The model under review builds one solid part; all positions refer to its coordinate system, in mm. A direction names the side the tool comes from. Round coordinates to 2 decimals unless told otherwise and drop trailing zeros. Order: outer loops, then holes, each group sorted by start corner. A loop starts at its lowest first (then second) coordinate and runs counter-clockwise, first axis right, second up. Notation, with made-up numbers: M -10,74.25 L 48,74.25 A27 ccw 48,100.25 Z; hole C 68,4 d11. An arc over 180 degrees is marked long. Answer as a JSON object with one key per item and string values. Group by question number.
1) Consider section A-A, the plane z = 0. Write out the cut boundary in (x, y), then the cut area to 3 significant figures.
2) For faces 1 (the flat face through (0, 26, 4.5)), 2 (the flat face through (1.05, 1, -5)), 3 (the flat face through (-0.1, 5, 18.2)), list the 3-axis set-ups (+Z, -Z, +X, -X, +Y, -Y) from which the entire face can be reached by the end or side of a thin tool; tool diameter is ignored.
3) Consider section B-B, the plane y = 16. Write out the cut boundary in (x, z), then the cut area to 3 significant figures.
4) Consider section C-C, the plane z = -14. Write out the cut boundary in (x, y).
5) The part is to be moulded in two halves that separate along Z. For faces 4 (the flat face through (6.5, 2.5, -19.5)), 5 (the cylindrical face through (0, 4, -18)), 6 (the flat face through (-6.5, 2.5, 19.5)), say which applies: +Z half, -Z half, draft (parallel to the pull), parting line (faces both ways), or undercut.
6) To check wall thickness, follow line 1 (Z direction, x = 0, y = 2.35); line 2 (Z direction, x = 0, y = 1.1); line 3 (Z direction, x = 0, y = 3.75). State the ranges of each line that lie inside material, in increasing order.
7) Insertion check: pin 1 Ø5.5 at (x, z) = (-1.5, -16) entering from +Y; pin 2 Ø1 at (x, z) = (0, -4.5) entering from -Y; pin 3 Ø1.5 at (x, y) = (0.5, 7) entering from +Z; pin 4 Ø4 at (x, z) = (0, 14) entering from +Y. Each pin has a flat end and moves straight along its axis. Give the tip position at first contact, or say it passes through.
Autodesk Inventor part; units mm, degrees
ref_plane "YZ Plane" through (0, 0, 0) normal (1, 0, 0) x (0, 1, 0)
ref_plane "XZ Plane" through (0, 0, 0) normal (0, 1, 0) x (-1, 0, 0)
ref_plane "XY Plane" through (0, 0, 0) normal (0, 0, 1) x (1, 0, 0)
sketch "Sketch1" plane through (0, 0, 0) normal (0, 1, 0) x (-1, 0, 0)
  line L0 (7, 9) -> (-7, 9)
  line L1 (-7, 9) -> (-7, -9)
  line L2 (-7, -9) -> (7, -9)
  line L3 (7, -9) -> (7, 9)
  line L4 (7, 9) -> (-7, -9) construction
  line L5 (-7, 9) -> (7, -9) construction
  point P0 (0, 0)
  dimension "POST_WIDTH" = 18
  dimension "POST_LENGTH" = 14
extrude "Extrusion1" add sketch "Sketch1" along normal blind 28.05
sketch "Sketch2" plane through (0, 0, 0) normal (0, -1, 0) x (1, 0, 0)
  line L0 (-7, -20) -> (7, -20)
  line L1 (7, -20) -> (7, 20)
  line L2 (7, 20) -> (-7, 20)
  line L3 (-7, 20) -> (-7, -20)
  line L4 (-7, -20) -> (7, 20) construction
  line L5 (7, -20) -> (-7, 20) construction
  line L6 (-7, -9) -> (-7, 9)
  line L7 (-7, 9) -> (7, 9)
  point P0 (0, 0)
  dimension "d4" = 0
  dimension "d5" = 11
extrude "Extrusion2" add sketch "Sketch2" against normal blind 5
sketch "Sketch3" plane through (0, 5, 0) normal (0, 1, 0) x (1, 0, 0)
  line L0 (-7, 20) -> (7, 20)
  line L1 (0, 20) -> (0, -20)
  line L2 (7, -20) -> (-7, -20)
  line L3 (7, -9) -> (7, 9)
  line L4 (7, 0) -> (-7, 0)
  line L5 (-7, 20) -> (-7, -20)
  point P0 (0, 0)
  point P1 (0, -14)
  point P2 (0, 14)
  dimension "d15" = 0
  dimension "d16" = 6
hole "Hole1" at (0, 5, 14) at (0, 5, -14) direction (0, -1, 0) diameter 4.5 end through all counterbore diameter 8 counterbore depth 2
chamfer "Chamfer2" distance 1 angle 45 2 edges at (0, 28.05, 9) (0, 28.05, -9)
sketch "Sketch8" plane through (7, 5, -9) normal (1, 0, 0) x (0, 0, -1)
  circle A0 centre (-9, 14.4933) radius 6.375
  circle A1 centre (-9, 14.4933) radius 6.883
  circle A2 centre (-10.8329, 9.4575) radius 1.524
  line L0 (-9, 14.4933) -> (-9, 7.6103)
  circle A3 centre (-7.1671, 9.4575) radius 1.524
  line L1 (-9, 14.4933) -> (-10.8329, 9.4575)
  line L2 (-18, 0) -> (-18, 22.05)
  line L3 (-17, 23.05) -> (-1, 23.05)
  circle A4 centre (-9, 14.05) radius 6
  line L4 (11, -5) -> (-29, -5)
  point P0 (-9, -5)
  point P1 (-6.6459, 8.0254)
  point P2 (-8.0195, 8.1942)
  point P3 (-12.2979, 9.0376)
  point P4 (-11.3541, 8.0254)
  point P5 (-5.7021, 9.0376)
  point P6 (-9.9805, 8.1942)
  dimension "d95" = 12
  dimension "HOLE_SIZE" = 12.75
  dimension "THREE_POINT_SIZE" = 13.766
  dimension "d51" = 3.048
  dimension "d52" = 20
  dimension "d55" = 9
  dimension "d96" = 19.05
extrude "Extrusion6" cut sketch "Sketch8" against normal up to surface (14 mm away) contours A0 A4 | A2 A0 | A4 A3 A0 L0 L1 A2 | A4 A2 | A0 A2 A4 | A4 A3 A0 | A0 A3 | A3 A4 | A2 L1 L0 A0 | A0 L0 A4 A2 | A2 A4 L0 A1 | A3 A4 L0 A0 | A1 L0 A4 A3
sketch "Sketch9" plane through (0, 28.05, 0) normal (0, 1, 0) x (1, 0, 0)
  line L0 (-7, 8) -> (-7, -8)
  line L1 (-7, -9) -> (7, -9)
  line L2 (7, -8) -> (7, 8)
  point P0 (0, 0)
  point P1 (-3.5, 0)
  point P2 (3.5, 0)
  dimension "d64" = 3.5
  dimension "d65" = 9
  dimension "d94" = 3.5
hole "Hole3" at (-3.5, 28.05, 0) at (3.5, 28.05, 0) direction (0, -1, 0) diameter 2.1565 end up to surface
chamfer "Chamfer3" distance 1 angle 45 4 edges at (7, 2.5, 20) (-7, 2.5, 20) (7, 2.5, -20) (-7, 2.5, -20)
sketch "Sketch10" plane through (0, 28.05, 0) normal (0, 1, 0) x (1, 0, 0)
  line L0 (-7, -9) -> (7, -9)
  line L1 (-1.75, -9) -> (1.75, -9)
  line L2 (1.75, -9) -> (1.75, -4.5)
  line L3 (1.75, -4.5) -> (-1.75, -4.5)
  line L4 (-1.75, -4.5) -> (-1.75, -9)
  line L5 (7, 9) -> (-7, 9)
  line L6 (-9.8, 0) -> (9.8, 0)
  line L7 (-1.75, 9) -> (1.75, 9)
  line L8 (1.75, 9) -> (1.75, 4.5)
  line L9 (1.75, 4.5) -> (-1.75, 4.5)
  line L10 (-1.75, 4.5) -> (-1.75, 9)
  point P0 (0, 0)
  point P1 (1.75, 5.6664)
  point P2 (1.75, 9)
  dimension "d71" = 4.5
  dimension "d72" = 3.5
  dimension "d73" = 1.75
extrude "Extrusion7" cut sketch "Sketch10" against normal blind 9
sketch "Sketch11" plane through (0, 0, 0) normal (0, -1, 0) x (1, 0, 0)
  line L0 (0, -4.5) -> (0, -5.5) construction
  line L1 (-1.05, -4.5) -> (-1.05, -5.5)
  line L2 (1.05, -5.5) -> (1.05, -4.5)
  arc A0 (1.05, -4.5) -> (-1.05, -4.5) centre (0, -4.5) ccw
  arc A1 (-1.05, -5.5) -> (1.05, -5.5) centre (0, -5.5) ccw
  point P0 (0, 0)
  point P1 (0, 5)
  point P2 (0, -5)
  dimension "d74" = 10
  dimension "d75" = 0
  dimension "d76" = 0
  dimension "d77" = 5
  dimension "d78" = 1.05
  dimension "d79" = 1
hole "Hole4" at (0, 0, 5) direction (0, 1, 0) diameter 2.1 depth 2.1
extrude "Extrusion8" cut sketch "Sketch11" against normal blind 2.1
sketch "Sketch12" plane through (-7, 5, 9) normal (-1, 0, 0) x (0, 0, 1)
  circle A0 centre (-9, -17.35) radius 12.7
  point P0 (-9, -5)
  dimension "d89" = 0
  dimension "d90" = 12.35
  dimension "d91" = 25.4
extrude "Extrusion9" cut sketch "Sketch12" against normal up to surface (14 mm away)
equation "\"HOLE_SIZE\" = 2 * HOLE_RADIUS + HOLE_TOLERANCE"
equation "\"d52\" = 0.5 * THREE_POINT_ANGLE"
equation "\"d71\" = 0.25 * POST_WIDTH"
equation "\"d72\" = 0.25 * POST_LENGTH"
equation "\"d69\" = EDGE_TO_HOLE"
equation "\"EDGE_TO_HOLE\" = POST_HEIGHT - BEAM_HEIGHT"
equation "\"BEAM_HEIGHT\" = 19.05"
equation "\"COLLIMATOR_DIAMETER\" = 12"
equation "\"THREE_POINT_ANGLE\" = 40deg"
equation "\"HOLE_RADIUS\" = 6.35"
equation "\"HOLE_TOLERANCE\" = 0.05"
properties part number "ADAPTER_collimator-BH19.05-D12.7"
Results list:
{
 "1": {"outline": "M -7,0.35 L 7,0.35 L 7,12.61 L -7,12.61 Z; M -7,25.87 L -4.58,25.87 L -4.58,28.05 L -7,28.05 Z; M -2.42,25.87 L 2.42,25.87 L 2.42,28.05 L -2.42,28.05 Z; M 4.58,25.87 L 7,25.87 L 7,28.05 L 4.58,28.05 Z", "area": "193 mm^2"},
 "2": {"face 1": "+Z, +Y", "face 2": "-Y", "face 3": "+Z, +X, -X, +Y"},
 "3": {"outline": "M -7,-9 L 7,-9 L 7,-5.33 L -7,-5.33 Z; M -7,5.33 L 7,5.33 L 7,9 L -7,9 Z", "area": "103 mm^2"},
 "4": {"outline": "M -7,0 L -2.25,0 L -2.25,3 L -4,3 L -4,5 L -7,5 Z; M 2.25,0 L 7,0 L 7,5 L 4,5 L 4,3 L 2.25,3 Z"},
 "5": {"face 4": "-Z half", "face 5": "undercut", "face 6": "+Z half"},
 "6": {"line 1": "-20 to -16.25, -11.75 to 11.75, 16.25 to 20", "line 2": "-20 to -16.25, -11.75 to -6.55, -3.45 to 3.95, 6.05 to 11.75, 16.25 to 20", "line 3": "-20 to -18, -10 to 10, 18 to 20"},
 "7": {"pin 1": "y = 5", "pin 2": "y = 2.1", "pin 3": "z = 9", "pin 4": "through"}
}
